from build123d import *

# Parameters (mm, degrees)
SKETCH1_W           = 60
SKETCH1_H           = 8
BOSS_EXTRUDE1_DEPTH = 1
SKETCH2_W           = 4.35
SKETCH2_H           = 7.6
BOSS_EXTRUDE2_DEPTH = 3
SKETCH3_R           = 1.17
CUT_EXTRUDE1_DEPTH  = 3
SKETCH4_W           = 7.92
SKETCH4_H           = 7.6
BOSS_EXTRUDE3_DEPTH = 1.93
SKETCH5_R           = 3.925
BOSS_EXTRUDE4_DEPTH = 3
SKETCH6_R           = 3.08
BOSS_EXTRUDE5_DEPTH = 4
SKETCH7_R           = 5
BOSS_EXTRUDE6_DEPTH = 3


with BuildPart() as part:
    # Sketch1 → Boss-Extrude1 (new body)
    with BuildSketch(Plane(origin=(0, 0, 0), x_dir=(1, 0, 0), z_dir=(0, 1, 0))):
        with Locations((30, -4)):
            Rectangle(SKETCH1_W, SKETCH1_H)
    extrude(amount=BOSS_EXTRUDE1_DEPTH)

    # Sketch2 → Boss-Extrude2 (add)
    with BuildSketch(Plane(origin=(0, 1, 0), x_dir=(1, 0, 0), z_dir=(0, 1, 0))):
        with Locations((57.625, -4)):
            Rectangle(SKETCH2_W, SKETCH2_H)
    extrude(amount=BOSS_EXTRUDE2_DEPTH)

    # Sketch3 → Cut-Extrude1 (cut)
    with BuildSketch(Plane(origin=(0, 1, 0), x_dir=(1, 0, 0), z_dir=(0, 1, 0))):
        with Locations(Location((52.38, -1.88, 0), (0, 0, 270))):
            Circle(SKETCH3_R)
        with Locations(Location((2.1, -6.12, 0), (0, 0, 270))):
            Circle(SKETCH3_R)
        with Locations(Location((2.1, -1.88, 0), (0, 0, 270))):
            Circle(SKETCH3_R)
    extrude(amount=-CUT_EXTRUDE1_DEPTH, mode=Mode.SUBTRACT)

    # Sketch4 → Boss-Extrude3 (add)
    with BuildSketch(Plane(origin=(0, 1, 0), x_dir=(1, 0, 0), z_dir=(0, 1, 0))):
        with Locations((32.54, -4)):
            Rectangle(SKETCH4_W, SKETCH4_H)
    extrude(amount=BOSS_EXTRUDE3_DEPTH)

    # Sketch5 → Boss-Extrude4 (add)
    with BuildSketch(Plane(origin=(0, 2.93, 0), x_dir=(1, 0, 0), z_dir=(0, 1, 0))):
        with Locations(Location((32.54, -4, 0), (0, 0, 75.50119591))):
            Circle(SKETCH5_R)
    extrude(amount=BOSS_EXTRUDE4_DEPTH)

    # Sketch6 → Boss-Extrude5 (add)
    with BuildSketch(Plane(origin=(0, 5.93, 0), x_dir=(1, 0, 0), z_dir=(0, 1, 0))):
        with Locations(Location((32.54, -4, 0), (0, 0, 270))):
            Circle(SKETCH6_R)
    extrude(amount=BOSS_EXTRUDE5_DEPTH)

    # Sketch7 → Boss-Extrude6 (add)
    with BuildSketch(Plane(origin=(0, 9.93, 0), x_dir=(1, 0, 0), z_dir=(0, 1, 0))):
        with Locations(Location((32.54, -4, 0), (0, 0, 270))):
            Circle(SKETCH7_R)
    extrude(amount=BOSS_EXTRUDE6_DEPTH)


solid = part.part
Build history of the part. All positions in model axes, mm. A direction names the side the tool comes from. Coordinates: 2 decimals unless noted, no trailing zeros. Order: outer loops, then holes, each group sorted by start corner. A loop starts at its lowest first (then second) coordinate and runs counter-clockwise, first axis right, second up. Notation, with made-up numbers: M 5.25,51 L 61.25,51 A15 ccw 61.25,73 Z; hole C 45.5,-23 d11. An arc over 180 degrees is marked long. One line per question, with ' | ' between items. Start each with the question number.
Q1. Probe L1, parallel to X at y = 0.6, z = 1.88; L2, parallel to X at y = 0.7, z = 6.12; L3, parallel to Y at x = 29, z = 1.5. List the from-to ranges inside material, lowest first. Write a range as from..to.
Q2. Flat gauge pins, fed straight in: pin 1 Ø3 at (y, z) = (10.5, 4) entering from -X; pin 2 Ø0.5 at (x, y) = (34, 0.5) entering from +Z; pin 3 Ø5 at (x, z) = (58, 2.5) entering from +Y; pin 4 Ø1.4 at (x, z) = (52.38, 1.88) entering from +Y. Where does each tip first touch, or does it go through?
Q3. 3-axis set-ups, long thin cutter, end or side, ignore diameter. For faces 4 (the face through (58, 2, 0.2)), 5 (the face through (37.497, 11.409, 3.349)), 6 (the face through (58, 4, 4)), 7 (the face through (35.594, 7.902, 3.599)): which of +Z, -Z, +X, -X, +Y, -Y reach the whole face in a straight line?
Q4. Saw through at C-C (x = 52.38). List the corners of the cut face in (y, z), then the cut area to 3 significant figures.
Q5. Saw through at A-A (x = 2.1). List the corners of the cut face in (y, z), then the cut area to 3 significant figures.
Q6. Two-plate mould, pull along Y, no slides. Class faces 1 (the face through (28.58, 2, 4)), 2 (the face through (58, 2, 7.8)), 3 (the face through (33, 12.93, 4)): +Y half, -Y half, draft (parallel to the pull), parting line (faces both ways), or undercut.
Q7. Saw through at D-D (y = 9.25). List the corners of the cut face in (x, z), then the cut area to 3 significant figures.
Q8. Saw through at B-B (z = 6.12). List the corners of the cut face in (x, y), then the cut area to 3 significant figures.
Check values:
1) L1: x = 0..0.93, 3.27..51.21, 53.55..60 | L2: x = 0..0.93, 3.27..60 | L3: y = 0..2.93, 9.93..12.93
2) pin 1: stops at x = 27.54 | pin 2: stops at z = 8 | pin 3: stops at y = 4 | pin 4: passes through
3) face 4: -Z, +X, +Y | face 5: +Y | face 6: +Z, -Z, +X, +Y | face 7: none
4) outline: M 0,0 L 1,0 L 1,0.71 L 0,0.71 Z; M 0,3.05 L 1,3.05 L 1,8 L 0,8 Z | area: 5.66 mm2
5) outline: M 0,0 L 1,0 L 1,0.71 L 0,0.71 Z; M 0,3.05 L 1,3.05 L 1,4.95 L 0,4.95 Z; M 0,7.29 L 1,7.29 L 1,8 L 0,8 Z | area: 3.32 mm2
6) face 1: undercut | face 2: draft | face 3: +Y half
7) outline: C 32.54,4 d6.16 | area: 29.8 mm2
8) outline: M 0,0 L 0.93,0 L 0.93,1 L 0,1 Z; M 3.27,0 L 60,0 L 60,1 L 59.8,1 L 59.8,4 L 55.45,4 L 55.45,1 L 36.5,1 L 36.5,2.93 L 35.84,2.93 L 35.84,5.93 L 34.77,5.93 L 34.77,9.93 L 37.07,9.93 L 37.07,12.93 L 28.01,12.93 L 28.01,9.93 L 30.31,9.93 L 30.31,5.93 L 29.24,5.93 L 29.24,2.93 L 28.58,2.93 L 28.58,1 L 3.27,1 Z | area: 151 mm2
